from build123d import *

# Parameters (mm, degrees)
SKETCH_1_R          = 2.72
EXTRUDE_4_DEPTH     = 28.26
CUT_EXTRUDE_1_DEPTH = 11.51
SKETCH_3_R          = 3.92
CUT_EXTRUDE_2_DEPTH = 10


with BuildPart() as part:
    # 草图1 → 凸台-拉伸4 (new body)
    with BuildSketch(Plane.XY):
        with BuildLine():
            Line((-34.509354159, -1.804921221), (-34.509354159, -38.304921221))
            Line((-34.509354159, -38.304921221), (23.530645841, -38.304921221))
            Line((23.530645841, -38.304921221), (23.530645841, -21.824921221))
            Line((23.530645841, -21.824921221), (-22.721234155, 4.232251332))
            ThreePointArc((-22.721234155, 4.232251332), (-30.46078359, 4.817148427), (-34.509354159, -1.804921221))
        make_face()
        with Locations((-27.069354159, -1.804921221)):
            Circle(SKETCH_1_R, mode=Mode.SUBTRACT)
    extrude(amount=EXTRUDE_4_DEPTH)

    # 草图2 → 切除-拉伸1 (cut, symmetric)
    with BuildSketch(Plane.XY.offset(14.13)):
        with BuildLine():
            Line((-35.9562977, -0.339763977), (-37.696904617, -35.707625719))
            Line((-37.696904617, -35.707625719), (23.935381019, -35.707625719))
            Line((23.935381019, -35.707625719), (23.935381019, -19.579879512))
            Line((23.935381019, -19.579879512), (-18.750112631, 5.187829847))
            ThreePointArc((-18.750112631, 5.187829847), (-29.978908557, 10.597270683), (-35.9562977, -0.339763977))
        make_face()
    extrude(amount=CUT_EXTRUDE_1_DEPTH, both=True, mode=Mode.SUBTRACT)

    # 草图3 → 切除-拉伸2 (cut)
    with BuildSketch(Plane(origin=(0, -35.707625719, 0), x_dir=(1, 0, 0), z_dir=(0, 1, 0))):
        with Locations(Location((12.530645841, -14.13, 0), (0, 0, 270))):
            Circle(SKETCH_3_R)
        with BuildLine():
            ThreePointArc((-26.319354159, -18.22), (-22.229354159, -14.13), (-26.319354159, -10.04))
            Line((-26.319354159, -10.04), (-34.509354159, -10.04))
            Line((-34.509354159, -10.04), (-34.509354159, -18.22))
            Line((-34.509354159, -18.22), (-26.319354159, -18.22))
        make_face()
    extrude(amount=-CUT_EXTRUDE_2_DEPTH, mode=Mode.SUBTRACT)


solid = part.part
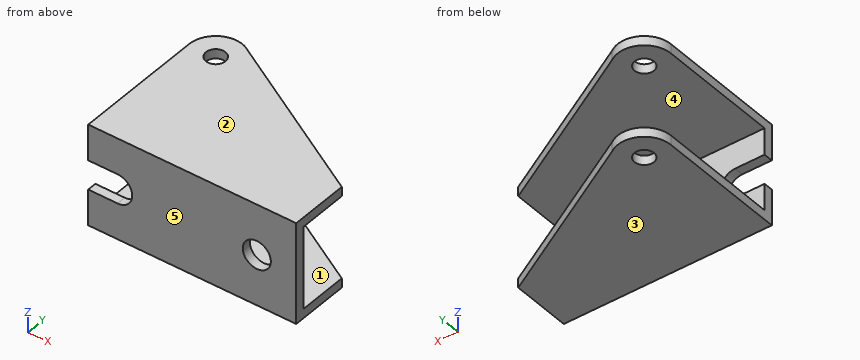
CAD build for the part. Positions are in the model's coordinates, mm. Face numbers are marked on the shaded views. A direction names the side the tool comes from. Give positions to 0.01 mm unless a question says otherwise; leave off trailing zeros. Loops run counter-clockwise (first coordinate to the right, second up) from the corner with the lowest first, then second, coordinate; pieces in that order, holes last. Notation, with made-up numbers: M -36.75,-13.75 L 9.25,-13.75 A31 cw 9.25,17.25 Z; hole C 32,80.5 d5. An arc over 180 degrees is marked long. One line per question, with ' | ' between items. Start each with the question number.
1. Saw through at D-D on x = 4. Give the cut face in (y, z).
2. Saw through at C-C on x = -27.5. Give the cut face in (y, z), plus the area to 3 significant figures.
3. Saw through at B-B on y = -34. Give the cut face in (x, z), plus the area to 3 significant figures.
4. Two-plate mould, pull along Z, no slides. Class the marked faces 1, 2 and 3: pulls with the +Z half, pulls with the -Z half, needs draft (parallel to the pull), parting line crosses it, or undercut.
5. Saw through at A-A on z = 14.13. Give the cut face in (x, y).
6. Flat gauge pin, fed straight in: pin 1 (1.3 mm diameter, centred on x = -31, y = -37.5, fed in from -Z). Where does the tip first touch, or does it go through?
7. Probe L1, parallel to Z at x = -11, y = -7; L2, parallel to Y at x = -27, z = 25; L3, parallel to Y at x = -30, z = 27.25. List the from-to ranges inside material, lowest first. Write a range as from..to.
8. 3-axis set-ups, long thin cutter, end or side, ignore diameter. For the marked faces 4 and 5: which of +Z, -Z, +X, -X, +Y, -Y reach the whole face in a straight line?
Result sheet:
1) outline: M -38.3,0 L -10.82,0 L -10.82,2.62 L -35.71,2.62 L -35.71,25.64 L -10.82,25.64 L -10.82,28.26 L -38.3,28.26 Z
2) outline: M -38.3,0 L -4.49,0 L -4.49,2.62 L -35.71,2.62 L -35.71,10.04 L -38.3,10.04 Z; M -38.3,18.22 L -35.71,18.22 L -35.71,25.64 L -4.49,25.64 L -4.49,28.26 L -38.3,28.26 Z; M 0.88,0 L 5.62,0 L 5.62,2.62 L 0.88,2.62 Z; M 0.88,25.64 L 5.62,25.64 L 5.62,28.26 L 0.88,28.26 Z | area: 241 mm^2
3) outline: M -34.51,0 L 23.53,0 L 23.53,2.62 L -34.51,2.62 Z; M -34.51,25.64 L 23.53,25.64 L 23.53,28.26 L -34.51,28.26 Z | area: 304 mm^2
4) face 1: undercut | face 2: pulls with the +Z half | face 3: pulls with the -Z half
5) outline: M -22.23,-38.3 L 8.61,-38.3 L 8.61,-35.71 L -22.23,-35.71 Z; M 16.45,-38.3 L 23.53,-38.3 L 23.53,-35.71 L 16.45,-35.71 Z
6) pin 1: stops at z = 0
7) L1: z = 0..2.62, 25.64..28.26 | L2: y = -38.3..-35.71 | L3: y = -38.3..5.03
8) face 4: +X, -X, +Y | face 5: +Z, -Z, +X, -X, -Y
